Check sheet for the modelled part. Datum: model origin and axes. Units: mm. A direction names the side the tool comes from. Round coordinates to 2 decimals unless told otherwise and drop trailing zeros. Order: outer loops, then holes, each group sorted by start corner. A loop starts at its lowest first (then second) coordinate and runs counter-clockwise, first axis right, second up.
```python
from build123d import *

# Parameters (mm, degrees)
F0_W     = 10
F0_H     = 30
F0_W_2   = 8
F0_H_2   = 15
F1_DEPTH = 15
F2_R     = 5


with BuildPart() as f1:
    # F0 (on Top) → F1 (new body)
    with BuildSketch(Plane.XY):
        with BuildLine():
            ThreePointArc((117, -13.1335928523), (184.6917420766, -0.6335928523), (117, 11.8664071477))
            Line((117, 11.8664071477), (117, -0.5232350183))
            Line((117, -0.5232350183), (117, -13.1335928523))
        make_face()
        with BuildLine():
            ThreePointArc((167.1917420766, -0.6335928523), (149.6622047421, -18.133567925), (132.1918417856, -0.5745182675))
            ThreePointArc((132.1918417856, -0.5745182675), (149.721279411, 16.8663822204), (167.1917420766, -0.6335928523))
        make_face(mode=Mode.SUBTRACT)
        Polygon((117, -0.5232350183), (-38, 0), (-38, -13.1335928523), (-28, -13.1335928523), (-18, -13.1335928523), (-10, -13.1335928523), (-6.7082043002, -13.1335928523), (6.7082043002, -13.1335928523), (117, -13.1335928523), align=None)
        Polygon((117, 11.8664071477), (-38, 11.8664071477), (-38, 0), (117, -0.5232350183), align=None)
        with BuildLine():
            ThreePointArc((167.1917420766, -0.6335928523), (149.721279411, 16.8663822204), (132.1918417856, -0.5745182675))
            ThreePointArc((132.1918417856, -0.5745182675), (149.6622047421, -18.133567925), (167.1917420766, -0.6335928523))
        make_face()
        with Locations((-33, -28.1335928523)):
            Rectangle(F0_W, F0_H)
        with Locations((-14, -20.6335928523)):
            Rectangle(F0_W_2, F0_H_2)
        Polygon((0, -26.5500005335), (6.7082043002, -13.1335928523), (-6.7082043002, -13.1335928523), align=None)
    extrude(amount=F1_DEPTH)

    # F2
    f2_edges = [f1.edges().sort_by_distance(p)[0] for p in [
        (39.5, 11.866407, 15),
        (61.854102, -13.133593, 15),
        (184.691742, -0.633593, 15),
        (-3.354102, -19.841797, 15),
        (-8.354102, -13.133593, 15),
        (-10, -20.633593, 15),
        (-33, -43.133593, 15),
        (-38, -15.633593, 15),
        (39.5, 11.866407, 0),
        (184.691742, -0.633593, 0),
        (61.854102, -13.133593, 0),
    ]]
    fillet(f2_edges, radius=F2_R)


solid = f1.part
```
Item 1: Scan lines: line 1 along X through (y, z) = (-18, 10.25) (3 decimals); line 2 along X through (y, z) = (-21.5, 1.75) (3 decimals); line 3 along Y through (x, z) = (112.5, 10). Record each from-to range of solid material in increasing order.
Answer:
line 1: x = -37.994 to -28, -18 to -10.006, -4.268 to 4.275, 119.311 to 180.072
line 2: x = -38 to -28, -18 to -10, -2.525 to 2.525, 123.102 to 176.281
line 3: y = -13.13 to 11.87
Item 2: Go/stop test with flat-tipped pins: P1, Ø2, axis at y = 12, z = 8.5, coming from the +X side; P2, Ø1.5, axis at x = 161.5, z = 4, coming from the -Y side; P3, Ø3, axis at x = 47, z = 5.5, coming from the -Y side. Record where each tip stops, or that it passes through.
Answer:
P1: stops at x = 182.7
P2: stops at y = -33.77
P3: stops at y = -13.13
Item 3: Sectioned sample at A-A (x = 54.5). Record the cut outline in (y, z).
Answer:
outline: (-13.13, 5) arc R5 ccw to (-8.13, 0) - (6.87, 0) arc R5 ccw to (11.87, 5) - (11.87, 10) arc R5 ccw to (6.87, 15) - (-8.13, 15) arc R5 ccw to (-13.13, 10) - close
Item 4: Access from +Z, -Z, +X, -X, +Y, -Y to the whole of each face (thin tool, end or side, straight path). Record for faces 4 (the flat face through (-18, -21, 7)), 5 (the cylindrical face through (64.474, -11.708, 1.504)), 6 (the cylindrical face through (-2.71, -17.94, 13.5)), 7 (the cylindrical face through (40.212, 10.441, 1.504)).
Answer:
face 4: +Z, -Z, -Y
face 5: -Z, -Y
face 6: +Z, -Y
face 7: -Z, -X, +Y
Item 5: Sectioned sample at B-B (z = 2.75). Record the cut outline in (x, y), and give its area (3 significant figures).
Answer:
outline: (-38, -43.13) - (-28, -43.13) - (-28, -13.13) - (-18, -13.13) - (-18, -28.13) - (-10, -28.13) - (-10, -13.13) - (-6.71, -13.13) - (0, -26.55) - (6.98, -12.6) - (117.37, -12.6) arc R34.47 ccw (long way) to (117.37, 11.33) - (-38, 11.33) - close
area: 7,950 mm2
Item 6: Release check for a two-part mould opening along X. For faces 1 (the flat face through (-28, -28, 7)), 2 (the cylindrical face through (40.212, 10.441, 13.496)), 3 (the cylindrical face through (-37, -16, 13)) record: released by +X, released by -X, zero draft, split by the parting line, or undercut.
Answer:
face 1: undercut
face 2: zero draft
face 3: released by -X
